The listing builds one solid part. Answer for the finished solid, in the listing's coordinates (mm). A direction names the side the tool comes from. Coordinates: 2 decimals unless noted, no trailing zeros. Order: outer loops, then holes, each group sorted by start corner. A loop starts at its lowest first (then second) coordinate and runs counter-clockwise, first axis right, second up. Notation, with made-up numbers: (58, 84) -> (86, 84) arc R27 cw to (86, 119) -> close; hole circle Ø3 at (61, 9.5). An arc over 180 degrees is marked (long way). Return JSON: item names as keys, results as strings.
from build123d import *

# Parameters (mm, degrees)
F0_W        = 10
F0_H        = 10
F1_DEPTH    = 3
F3_DEPTH    = 10
F4_T1_DEPTH = 10


# Not quite as in the source:
# - a fillet or chamfer that OpenCascade refuses, or shapes differently, is made with other operations: its cross-section is extruded or revolved along the edge and cut away or added


with BuildPart() as f1:
    # F0 (on Top) → F1 (new body)
    with BuildSketch(Plane.XY):
        Rectangle(F0_W, F0_H)
    extrude(amount=-F1_DEPTH)

    # F2 (on face) → F3 (join)
    with BuildSketch(Plane(origin=(0, 5, 0), x_dir=(-1, 0, 0), z_dir=(0, 1, 0))):
        with BuildLine():
            Line((0, -0.9684120044), (0, -2.9684120044))
            ThreePointArc((0, -2.9684120044), (3.9773759731, 5.0615187488), (-4.8204695111, 3.359395848))
            Line((-4.8204695111, 3.359395848), (-2.8922817066, 2.828272707))
            ThreePointArc((-2.8922817066, 2.828272707), (2.3864255838, 3.8495464475), (0, -0.9684120044))
        make_face()
    extrude(amount=-F3_DEPTH)

    # F4: fillet of radius 5 on 1 edges, made by hand

    # F4_s2 → F4_t1 (join)
    with BuildSketch(Plane.XZ.offset(-5)):
        with BuildLine():
            ThreePointArc((-5, 0), (-4.930361996, 0.7167697097), (-4.9644138164, 1.4361088104))
            ThreePointArc((-4.9644138164, 1.4361088104), (-4.8203188847, 0.7032334307), (-4.5686595645, 0))
            Line((-4.5686595645, 0), (-5, 0))
        make_face()
    extrude(amount=F4_T1_DEPTH)


solid = f1.part
1. The part is cut by section C-C on z = 2. Give the vertices of the cut face in (x, y), and give its area (3 significant figures).
Answer block:
{"outline": "(-5, -5) -> (-3, -5) -> (-3, 5) -> (-5, 5) -> close", "area": "20.0 mm2"}
2. Each of these flat-tipped pins is pushed along its axis until it touches: pin 1 Ø3 at (x, y) = (3, 2) entering from +Z; pin 2 Ø2 at (x, z) = (0, 3) entering from +Y; pin 3 Ø2 at (x, y) = (3.5, 0) entering from +Z. Where does it stop, or does it pass through?
Answer block:
{"pin 1": "stops at z = 6.8", "pin 2": "passes through", "pin 3": "stops at z = 6.36"}
3. Consider line 1 (Z direction, x = 0, y = 1); line 2 (Z direction, x = 3, y = 3.5); line 3 (X direction, y = -1.25, z = 4). Determine where each line is inside the solid, lowest interval first. Write a range as from..to.
Answer block:
{"line 1": "z = -3..0, 5.03..7.03", "line 2": "z = -3..0, 2.86..6.03", "line 3": "x = -4.6..-2.26, 2.26..4.6"}
4. The part is cut by section B-B on y = 3. Give the vertices of the cut face in (x, z), and give its area (3 significant figures).
Answer block:
{"outline": "(-5, -3) -> (5, -3) -> (5, 0) -> (-2.21, 0) arc R3 cw (long way) to (2.89, 2.83) -> (4.82, 3.36) arc R5 ccw to (-4.96, 1.44) arc R5 cw to (-5, 0) -> close", "area": "57.5 mm2"}
5. The part is cut by section A-A on x = 0. Give the vertices of the cut face in (y, z), and give its area (3 significant figures).
Answer block:
{"outline": "(-5, -3) -> (5, -3) -> (5, 0) -> (-5, 0) -> close; (-5, 5.03) -> (5, 5.03) -> (5, 7.03) -> (-5, 7.03) -> close", "area": "50.0 mm2"}
6. For faces 1 (the face through (1, 0, 0)), 2 (the face through (-1.39, 0.07, 4.69)), determine the directions among +Z, -Z, +X, -X, +Y, -Y from which every point of the face is accessible in a straight line to the end or side of a thin tool.
Answer block:
{"face 1": "+X, +Y, -Y", "face 2": "+Y, -Y"}
7. The part is cut by section D-D on z = 5.5. Give the vertices of the cut face in (x, y).
Answer block:
{"outline": "(-3.6, -5) -> (3.6, -5) -> (3.6, 5) -> (-3.6, 5) -> close"}
8. Determine the mould class of faces 3 (the face through (0, 5, -1)), 4 (the face through (3.87, 0.07, 3.098)), 5 (the face through (0, 0, -3)) for opening direction Z: pulls with the +Z half, pulls with the -Z half, needs draft (parallel to the pull), parting line crosses it, or undercut.
Answer block:
{"face 3": "needs draft", "face 4": "undercut", "face 5": "pulls with the -Z half"}
